Read the model definition and answer for the solid it produces. Units are mm, in the model's axes. A direction names the side the tool comes from. Coordinates: 2 decimals unless noted, no trailing zeros. Loops run counter-clockwise (first coordinate to the right, second up) from the corner with the lowest first, then second, coordinate; pieces in that order, holes last.
Q1. Flat-ended cylindrical pins translate along their axes: P1, Ø1, axis at x = -101, z = 385.5, coming from the -Y side; P2, Ø3, axis at y = 119, z = 271.5, coming from the -X side. Find the tip coordinate at first contact, or state that the pin passes through.
Q2. Section A-A (z = 499.5) is taken. Give the vertices of the cut face in (x, y).
Q3. Which of the six approach directions +Z, -Z, +X, -X, +Y, -Y give full straight-line access (tool end or side, diameter ignored) to faces 4 (the face through (283, 0, 386)), 5 (the face through (-114.993, 189, 385)), 6 (the face through (61, 6.35, 385))?
Q4. The mould has two halves that part along Z. Classify faces 1 (the face through (558.107, 185, 376)), 2 (the face through (392, 6.35, 385)), 3 (the face through (223, 190, 0)): pulls with the +Z half, pulls with the -Z half, needs draft (parallel to the pull), parting line crosses it, or undercut.
Q5. Straight lines are drawn through the part: line 1 (X direction, y = 293, z = 176.5); line 2 (Y direction, x = 111.5, z = 107). For each, find the intervals that lie inside material, in ascending order.
from build123d import *

# Parameters (mm, degrees)
F0_W     = 327.025
F0_H     = 762
F0_W_2   = 203.2
F0_H_2   = 635
F0_W_3   = 324.993
F0_W_4   = 3.175
F0_W_5   = 2.032
F1_DEPTH = 374.65
F2_DEPTH = 6.35
F3_W     = 368.3
F3_H     = 762
F3_W_2   = 247.65
F3_H_2   = 635
F3_W_3   = 6.35
F4_DEPTH = 19.05
F5_DEPTH = 12.7


# Not quite as in the source:
# - a feature names something its author has since deleted; it is built from what else it names


with BuildPart() as f1:
    # F0 (on Front) → F1 (new body)
    with BuildSketch(Plane.XZ):
        with Locations((394.5947425127, 381)):
            Rectangle(F0_W, F0_H)
        with Locations((393.0072425127, 381)):
            Rectangle(F0_W_2, F0_H_2, mode=Mode.SUBTRACT)
        with Locations((62.2357425127, 381)):
            Rectangle(F0_W_3, F0_H)
        with Locations((62.8072425127, 381)):
            Rectangle(F0_W_2, F0_H_2, mode=Mode.SUBTRACT)
        with Locations((62.8072425127, 381)):
            Rectangle(F0_W_2, F0_H_2)
        with Locations((393.0072425127, 381)):
            Rectangle(F0_W_2, F0_H_2)
        with Locations((226.3197425127, 381)):
            Rectangle(F0_W_4, F0_H)
        with Locations((229.4947425127, 381)):
            Rectangle(F0_W_4, F0_H)
        with Locations((-101.2767574873, 381)):
            Rectangle(F0_W_5, F0_H)
    extrude(amount=-F1_DEPTH)

    # F0 (on Front) → F2 (cut)
    with BuildSketch(Plane.XZ):
        with Locations((226.3197425127, 381)):
            Rectangle(F0_W_4, F0_H)
        with Locations((229.4947425127, 381)):
            Rectangle(F0_W_4, F0_H)
        with Locations((-101.2767574873, 381)):
            Rectangle(F0_W_5, F0_H)
        with Locations((62.8072425127, 381)):
            Rectangle(F0_W_2, F0_H_2)
        with Locations((393.0072425127, 381)):
            Rectangle(F0_W_2, F0_H_2)
    extrude(amount=-F2_DEPTH, mode=Mode.SUBTRACT)

    # F3 (on face) → F4 (join)
    with BuildSketch(Plane(origin=(-102.2927574873, 0, 0), x_dir=(0, -1, 0), z_dir=(-1, 0, 0))):
        with Locations((-190.5, 381)):
            Rectangle(F3_W, F3_H)
        with Locations((-187.325, 381)):
            Rectangle(F3_W_2, F3_H_2, mode=Mode.SUBTRACT)
        with Locations((-3.175, 381)):
            Rectangle(F3_W_3, F3_H)
    extrude(amount=F4_DEPTH)

    # F3 (on face) → F5 (join)
    with BuildSketch(Plane(origin=(-102.2927574873, 0, 0), x_dir=(0, -1, 0), z_dir=(-1, 0, 0))):
        with Locations((-187.325, 381)):
            Rectangle(F3_W_2, F3_H_2)
    extrude(amount=F5_DEPTH)


solid = f1.part
Numbers:
1. P1: stops at y = 6.35
1. P2: stops at x = -114.99
2. outline: (-121.34, 0) - (-102.29, 0) - (-102.29, 6.35) - (-100.26, 6.35) - (-100.26, 0) - (-38.79, 0) - (-38.79, 6.35) - (164.41, 6.35) - (164.41, 0) - (224.73, 0) - (224.73, 6.35) - (231.08, 6.35) - (231.08, 0) - (291.41, 0) - (291.41, 6.35) - (494.61, 6.35) - (494.61, 0) - (558.11, 0) - (558.11, 374.65) - (-121.34, 374.65) - (-121.34, 311.15) - (-114.99, 311.15) - (-114.99, 63.5) - (-121.34, 63.5) - close
3. face 4: +Z, -Z, +X, -X, -Y
3. face 5: -X
3. face 6: -Y
4. face 1: needs draft
4. face 2: undercut
4. face 3: pulls with the -Z half
5. line 1: x = -114.99 to 558.11
5. line 2: y = 6.35 to 374.65
